The listing builds one solid part. Answer for the finished solid, in the listing's coordinates (mm). A direction names the side the tool comes from. Round coordinates to 2 decimals unless told otherwise and drop trailing zeros. Write each loop counter-clockwise with the first axis right and the second up, starting at its lowest first coordinate (ties: lowest second). Pieces come first, ordered by that corner, then holes. Notation, with made-up numbers: (-6, -29) - (14, -29) arc R31 cw to (14, 1) - close; hole circle Ø7 at (72, 74.25). An arc over 180 degrees is marked (long way). Answer in a Markdown table with one row per item.
from build123d import *

# Parameters (mm, degrees)
SKETCH1_W           = 100
SKETCH1_H           = 72.907808631
SKETCH1_R           = 2
SKETCH1_R_2         = 2.083080247
BOSS_EXTRUDE1_DEPTH = 4
BOSS_EXTRUDE2_DEPTH = 100
SKETCH3_R           = 2.5
CUT_EXTRUDE1_DEPTH  = 4
SKETCH4_W           = 54.032487287
SKETCH4_H           = 4.238299892
SKETCH4_W_2         = 12.902793756
CUT_EXTRUDE4_DEPTH  = 2


with BuildPart() as part:
    # Sketch1 → Boss-Extrude1 (new body)
    with BuildSketch(Plane(origin=(0, 0, 0), x_dir=(1, 0, 0), z_dir=(0, 1, 0))):
        with Locations((50, 36.453904316)):
            Rectangle(SKETCH1_W, SKETCH1_H)
        with Locations((97.5, 70.407808631)):
            Circle(SKETCH1_R, mode=Mode.SUBTRACT)
        with Locations((2.5, 38)):
            Circle(SKETCH1_R, mode=Mode.SUBTRACT)
        with Locations((82.5, 3.5)):
            Circle(SKETCH1_R, mode=Mode.SUBTRACT)
        with Locations((20, 3.5)):
            Circle(SKETCH1_R_2, mode=Mode.SUBTRACT)
    extrude(amount=BOSS_EXTRUDE1_DEPTH)

    # Sketch2 → Boss-Extrude2 (add)
    with BuildSketch(Plane.ZY):
        with BuildLine():
            Line((0, 4), (5, 4))
            Line((5, 4), (5, 29))
            Line((5, 29), (9, 29))
            Line((9, 29), (9, 5.38521522))
            Line((9, 5.38521522), (9, 4))
            ThreePointArc((9, 4), (7.828427125, 1.171572875), (5, 0))
            Line((5, 0), (0, 0))
            Line((0, 0), (0, 4))
        make_face()
    extrude(amount=-BOSS_EXTRUDE2_DEPTH)

    # Sketch3 → Cut-Extrude1 (cut)
    with BuildSketch(Plane.XY.offset(9)):
        with Locations((15, 16.5)):
            Circle(SKETCH3_R)
        with Locations((85, 16.5)):
            Circle(SKETCH3_R)
    extrude(amount=-CUT_EXTRUDE1_DEPTH, mode=Mode.SUBTRACT)

    # Sketch4 → Cut-Extrude4 (cut)
    with BuildSketch(Plane.XZ):
        Polygon((51.950078291, -63.631079916), (12.647642859, -63.631079916), (12.647642859, -44.280868197), (3.432980611, -44.280868197), (3.432980611, -70.907808631), (12.647642859, -70.907808631), (91.252513722, -70.907808631), (97.892827947, -63.631079916), (97.892827947, -36.415165299), (91.252513722, -36.415165299), (91.252513722, -63.631079916), (61.978819372, -63.631079916), (61.978819372, -54.74747752), (51.950078291, -54.74747752), align=None)
        with Locations((51.441944052, -3.540646856)):
            Rectangle(SKETCH4_W, SKETCH4_H)
        with Locations((9.884377489, -3.540646856)):
            Rectangle(SKETCH4_W_2, SKETCH4_H)
    extrude(amount=-CUT_EXTRUDE4_DEPTH, mode=Mode.SUBTRACT)


solid = part.part
(1) For faces 4 (the flat face through (78.458, 1, -4)), 5 (the cylindrical face through (84.408, 1.972, -4.101)), 6 (the flat face through (49, 4, -34)), determine the directions among +Z, -Z, +X, -X, +Y, -Y from which every point of the face is accessible in a straight line to the end or side of a thin tool.
Checked values:
| item | result |
|---|---|
| face 4 | -Y |
| face 5 | +Y, -Y |
| face 6 | -Z, +X, -X, +Y |
(2) Section D-D (z = -42) is taken. Give the vertices of the cut face in (x, y).
Checked values:
| item | result |
|---|---|
| outline | (0, 0) - (91.25, 0) - (91.25, 2) - (97.89, 2) - (97.89, 0) - (100, 0) - (100, 4) - (0, 4) - close |
(3) Section A-A (x = 20) is taken. Give the vertices of the cut face in (y, z).
Checked values:
| item | result |
|---|---|
| outline | (0, -72.91) - (4, -72.91) - (4, -5.58) - (0, -5.58) - (0, -63.63) - (2, -63.63) - (2, -70.91) - (0, -70.91) - close; (0, -1.42) - (4, -1.42) - (4, 5) - (29, 5) - (29, 9) - (4, 9) arc R4 ccw to (0, 5) - close |
(4) For a pull along X with two mould halves and no side action, classify faces 1 (the cylindrical face through (49.3, 1.203, 7.859)), 2 (the flat face through (51, 2, -4)), 3 (the flat face through (100, 3.8, -25.7)) as pulls with the +X half, pulls with the -X half, needs draft (parallel to the pull), parting line crosses it, or undercut.
Checked values:
| item | result |
|---|---|
| face 1 | needs draft |
| face 2 | undercut |
| face 3 | pulls with the +X half |
(5) Flat-ended cylindrical pins translate along their axes: pin 1 (23.5 mm diameter, centred on x = 55, z = -44.5, fed in from +Y); pin 2 (1.6 mm diameter, centred on x = 46.5, y = 1.5, fed in from +Z); pin 3 (2 mm diameter, centred on x = 75, y = 25, fed in from -Z). Find the tip coordinate at first contact, or state that the pin passes through.
Checked values:
| item | result |
|---|---|
| pin 1 | stops at y = 4 |
| pin 2 | stops at z = 8.62 |
| pin 3 | stops at z = 5 |
(6) Section C-C (x = 56) is taken. Give the vertices of the cut face in (y, z), and give its area (3 significant figures).
Checked values:
| item | result |
|---|---|
| outline | (0, -72.91) - (4, -72.91) - (4, 5) - (29, 5) - (29, 9) - (4, 9) arc R4 ccw to (0, 5) - (0, -1.42) - (2, -1.42) - (2, -5.66) - (0, -5.66) - (0, -54.75) - (2, -54.75) - (2, -70.91) - (0, -70.91) - close |
| area | 383 mm2 |
(7) Section B-B (y = 16.5) is taken. Give the vertices of the cut face in (x, z).
Checked values:
| item | result |
|---|---|
| outline | (0, 5) - (12.5, 5) - (12.5, 9) - (0, 9) - close; (17.5, 5) - (82.5, 5) - (82.5, 9) - (17.5, 9) - close; (87.5, 5) - (100, 5) - (100, 9) - (87.5, 9) - close |
(8) Find the intervals of material crossed by line 1 (Z direction, x = 82.5, y = 1.4); line 2 (Z direction, x = 20, y = 1.65); line 3 (Z direction, x = 54, y = 22.25), in increasing order.
Checked values:
| item | result |
|---|---|
| line 1 | z = -72.91 to -70.91, -63.63 to -5.5, -1.5 to 8.04 |
| line 2 | z = -72.91 to -70.91, -63.63 to -5.58, -1.42 to 8.24 |
| line 3 | z = 5 to 9 |
